Input: part model. Units: mm. Frame: model coordinates. A direction names the side the tool comes from. Round coordinates to 2 decimals unless told otherwise and drop trailing zeros. Order: outer loops, then holes, each group sorted by start corner. A loop starts at its lowest first (then second) coordinate and runs counter-clockwise, first axis right, second up. Notation, with made-up numbers: (38.5, 76) -> (50.5, 76) arc R11 cw to (50.5, 95) -> close; hole circle Ø1 at (45.25, 57). An arc over 180 degrees is marked (long way). Use a Markdown table: item, result.
from build123d import *

# Parameters (mm, degrees)
SKETCH1_R           = 2.3
BOSS_EXTRUDE1_DEPTH = 5
BOSS_EXTRUDE2_DEPTH = 9
BOSS_EXTRUDE3_DEPTH = 0.9
FILLET2_R           = 0.1


with BuildPart() as part:
    # Sketch1 → Boss-Extrude1 (new body)
    with BuildSketch(Plane(origin=(0, 0, 0), x_dir=(1, 0, 0), z_dir=(0, 1, 0))):
        Circle(SKETCH1_R)
    extrude(amount=BOSS_EXTRUDE1_DEPTH)

    # Sketch2 → Boss-Extrude2 (add)
    with BuildSketch(Plane(origin=(0, 5, 0), x_dir=(1, 0, 0), z_dir=(0, 1, 0))):
        with BuildLine():
            Line((0.05, 3.55), (-0.05, 3.55))
            ThreePointArc((-0.05, 3.55), (-0.580330086, 3.330330086), (-0.8, 2.8))
            Line((-0.8, 2.8), (-0.8, 2.891366459))
            ThreePointArc((-0.8, 2.891366459), (-2.121320344, 2.121320344), (-2.891366459, 0.8))
            Line((-2.891366459, 0.8), (-2.8, 0.8))
            ThreePointArc((-2.8, 0.8), (-3.330330086, 0.580330086), (-3.55, 0.05))
            Line((-3.55, 0.05), (-3.55, -0.05))
            ThreePointArc((-3.55, -0.05), (-3.330330086, -0.580330086), (-2.8, -0.8))
            Line((-2.8, -0.8), (-2.891366459, -0.8))
            ThreePointArc((-2.891366459, -0.8), (-2.121320344, -2.121320344), (-0.8, -2.891366459))
            Line((-0.8, -2.891366459), (-0.8, -2.8))
            ThreePointArc((-0.8, -2.8), (-0.580330086, -3.330330086), (-0.05, -3.55))
            Line((-0.05, -3.55), (0.05, -3.55))
            ThreePointArc((0.05, -3.55), (0.580330086, -3.330330086), (0.8, -2.8))
            Line((0.8, -2.8), (0.8, -2.891366459))
            ThreePointArc((0.8, -2.891366459), (2.121320344, -2.121320344), (2.891366459, -0.8))
            Line((2.891366459, -0.8), (2.8, -0.8))
            ThreePointArc((2.8, -0.8), (3.330330086, -0.580330086), (3.55, -0.05))
            Line((3.55, -0.05), (3.55, 0.05))
            ThreePointArc((3.55, 0.05), (3.330330086, 0.580330086), (2.8, 0.8))
            Line((2.8, 0.8), (2.891366459, 0.8))
            ThreePointArc((2.891366459, 0.8), (2.121320344, 2.121320344), (0.8, 2.891366459))
            Line((0.8, 2.891366459), (0.8, 2.8))
            ThreePointArc((0.8, 2.8), (0.580330086, 3.330330086), (0.05, 3.55))
        make_face()
    extrude(amount=BOSS_EXTRUDE2_DEPTH)

    # Sketch3 → Boss-Extrude3 (add)
    with BuildSketch(Plane(origin=(0, 14, 0), x_dir=(1, 0, 0), z_dir=(0, 1, 0))):
        with BuildLine():
            Line((-0.4, 1.35), (0.4, 1.35))
            ThreePointArc((0.4, 1.35), (0.576776695, 1.276776695), (0.65, 1.1))
            Line((0.65, 1.1), (0.65, 0.9))
            ThreePointArc((0.65, 0.9), (0.723223305, 0.723223305), (0.9, 0.65))
            Line((0.9, 0.65), (1.1, 0.65))
            ThreePointArc((1.1, 0.65), (1.276776695, 0.576776695), (1.35, 0.4))
            Line((1.35, 0.4), (1.35, -0.4))
            ThreePointArc((1.35, -0.4), (1.276776695, -0.576776695), (1.1, -0.65))
            Line((1.1, -0.65), (0.9, -0.65))
            ThreePointArc((0.9, -0.65), (0.723223305, -0.723223305), (0.65, -0.9))
            Line((0.65, -0.9), (0.65, -1.1))
            ThreePointArc((0.65, -1.1), (0.576776695, -1.276776695), (0.4, -1.35))
            Line((0.4, -1.35), (-0.4, -1.35))
            ThreePointArc((-0.4, -1.35), (-0.576776695, -1.276776695), (-0.65, -1.1))
            Line((-0.65, -1.1), (-0.65, -0.9))
            ThreePointArc((-0.65, -0.9), (-0.723223305, -0.723223305), (-0.9, -0.65))
            Line((-0.9, -0.65), (-1.1, -0.65))
            ThreePointArc((-1.1, -0.65), (-1.276776695, -0.576776695), (-1.35, -0.4))
            Line((-1.35, -0.4), (-1.35, 0.4))
            ThreePointArc((-1.35, 0.4), (-1.276776695, 0.576776695), (-1.1, 0.65))
            Line((-1.1, 0.65), (-0.9, 0.65))
            ThreePointArc((-0.9, 0.65), (-0.723223305, 0.723223305), (-0.65, 0.9))
            Line((-0.65, 0.9), (-0.65, 1.1))
            ThreePointArc((-0.65, 1.1), (-0.576776695, 1.276776695), (-0.4, 1.35))
        make_face()
    extrude(amount=BOSS_EXTRUDE3_DEPTH)

    # Fillet2
    fillet2_edges = [part.edges().sort_by_distance(p)[0] for p in [
        (0.723223305, 14.9, 0.723223305),
        (1, 14.9, 0.65),
        (1.276776695, 14.9, 0.576776695),
        (1.35, 14.9, 0),
        (1.276776695, 14.9, -0.576776695),
        (1, 14.9, -0.65),
        (0.723223305, 14.9, -0.723223305),
        (0.65, 14.9, -1),
        (0.576776695, 14.9, -1.276776695),
        (0, 14.9, -1.35),
        (-0.576776695, 14.9, -1.276776695),
        (-0.65, 14.9, -1),
        (-0.723223305, 14.9, -0.723223305),
        (-1, 14.9, -0.65),
        (-1.276776695, 14.9, -0.576776695),
        (-1.35, 14.9, 0),
        (-1.276776695, 14.9, 0.576776695),
        (-1, 14.9, 0.65),
        (-0.723223305, 14.9, 0.723223305),
        (-0.65, 14.9, 1),
        (-0.576776695, 14.9, 1.276776695),
        (0, 14.9, 1.35),
        (0.576776695, 14.9, 1.276776695),
        (0.65, 14.9, 1),
    ]]
    fillet(fillet2_edges, radius=FILLET2_R)


solid = part.part
1) Pin query (flat end, axial travel): pin 1 Ø1.5 at (y, z) = (1.5, -1) entering from -X; pin 2 Ø0.9 at (x, y) = (0, 14.5) entering from -Z; pin 3 Ø3 at (x, z) = (2.5, -2.5) entering from +Y. Return the tip coordinate at first contact, or that it passes through.
Results found:
| item | result |
|---|---|
| pin 1 | stops at x = -2.29 |
| pin 2 | stops at z = -1.35 |
| pin 3 | stops at y = 14 |
2) Line query: L1, parallel to Y at x = 1.25, z = -0.75; L2, parallel to Y at x = -2.25, z = 1; L3, parallel to Z at x = 0.25, y = 1.75. Output: solid intervals per line, ascending. Write a range as [from, to].
Results found:
| item | result |
|---|---|
| L1 | y = [0, 14] |
| L2 | y = [5, 14] |
| L3 | z = [-2.29, 2.29] |
3) Cut plane A-A on y = 10.75. Return loops of the section in (x, z), and give its area (3 significant figures).
Results found:
| item | result |
|---|---|
| outline | (-3.55, -0.05) arc R0.75 ccw to (-2.8, -0.8) -> (-2.89, -0.8) arc R3 ccw to (-0.8, -2.89) -> (-0.8, -2.8) arc R0.75 ccw to (-0.05, -3.55) -> (0.05, -3.55) arc R0.75 ccw to (0.8, -2.8) -> (0.8, -2.89) arc R3 ccw to (2.89, -0.8) -> (2.8, -0.8) arc R0.75 ccw to (3.55, -0.05) -> (3.55, 0.05) arc R0.75 ccw to (2.8, 0.8) -> (2.89, 0.8) arc R3 ccw to (0.8, 2.89) -> (0.8, 2.8) arc R0.75 ccw to (0.05, 3.55) -> (-0.05, 3.55) arc R0.75 ccw to (-0.8, 2.8) -> (-0.8, 2.89) arc R3 ccw to (-2.89, 0.8) -> (-2.8, 0.8) arc R0.75 ccw to (-3.55, 0.05) -> close |
| area | 31.1 mm² |
4) Set-up query: faces 1 (the flat face through (1, 14, -1)), 2 (the cylindrical face through (2.137, 9.437, -2.106)), 3 (the cylindrical face through (-1.825, 2.465, 1.4)). Return all of +Z, -Z, +X, -X, +Y, -Y with unobstructed straight access to the full face (end or side cutting, diameter ignored); none if empty.
Results found:
| item | result |
|---|---|
| face 1 | +Y |
| face 2 | -Z, +X, +Y, -Y |
| face 3 | -Y |
5) Cut plane B-B on z = -0.25. Return loops of the section in (x, y), and give its area (3 significant figures).
Results found:
| item | result |
|---|---|
| outline | (-3.52, 5) -> (-2.29, 5) -> (-2.29, 0) -> (2.29, 0) -> (2.29, 5) -> (3.52, 5) -> (3.52, 14) -> (1.35, 14) -> (1.35, 14.8) arc R0.1 ccw to (1.25, 14.9) -> (-1.25, 14.9) arc R0.1 ccw to (-1.35, 14.8) -> (-1.35, 14) -> (-3.52, 14) -> close |
| area | 88.7 mm² |
6) Cut plane D-D on y = 2. Return loops of the section in (x, z), and give its area (3 significant figures).
Results found:
| item | result |
|---|---|
| outline | circle Ø4.6 at (0, 0) |
| area | 16.6 mm² |
7) Cut plane C-C on x = -1.5. Return loops of the section in (y, z).
Results found:
| item | result |
|---|---|
| outline | (0, -1.74) -> (5, -1.74) -> (5, -2.6) -> (14, -2.6) -> (14, 2.6) -> (5, 2.6) -> (5, 1.74) -> (0, 1.74) -> close |
